Geometry: see drawing. Coordinates: mm, zero at the bounding-box minimum. A direction names the side the tool comes from. Coordinates: 2 decimals unless noted, no trailing zeros. Loops run counter-clockwise (first coordinate to the right, second up) from the corner with the lowest first, then second, coordinate; pieces in that order, holes last. Notation, with made-up numbers: (-26.5, 60) -> (11.5, 60) arc R25 ccw to (11.5, 80) -> close; hole circle Ø4 at (35, 16.5). An arc over 180 degrees is marked (long way). One line per item, written item: value. Start each with the question number.
Item 1: Set-up query: the marked faces 1, 2 and 3. Return all of +Z, -Z, +X, -X, +Y, -Y with unobstructed straight access to the full face (end or side cutting, diameter ignored); none if empty.
Item 2: Contact query for flat-ended pins moving along their axis: pin 1 Ø8 at (y, z) = (20, 15) entering from +X; pin 2 Ø2 at (x, z) = (54.5, 16) entering from +Y; pin 3 Ø6 at (y, z) = (36.5, 6) entering from +X; pin 4 Ø10 at (x, y) = (45, 14) entering from -Z. Output: stop coordinate, or through.
Item 3: Section query A-A on x = 10. Return loops of the section in (y, z), then the cut area to 3 significant figures.
Item 4: Section query D-D on x = 95.5. Return loops of the section in (y, z).
Item 5: Section query B-B on z = 3.25. Return loops of the section in (x, y), then the cut area to 3 significant figures.
Item 6: Section query C-C on z = 10. Return loops of the section in (x, y), then the cut area to 3 significant figures.
Item 7: Ray query, probe 1 along Z at (x, y) = (10, 1); probe 2 along Y at (x, z) = (13.5, 13.75); probe 3 along Y at (x, z) = (39, 14) (1 decimal). Return the intervals inside material, ascending. Write a range as from..to.
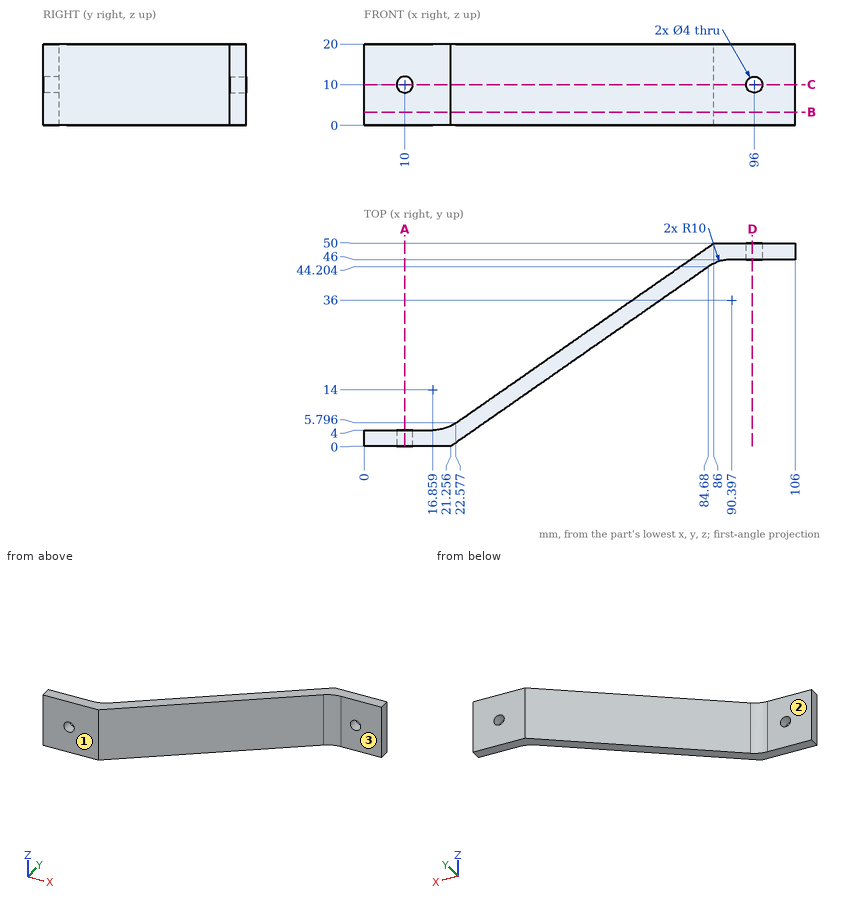
Reply:
1. face 1: +Z, -Z, +X, -X, -Y
1. face 2: +Z, -Z, -X, +Y
1. face 3: +Z, -Z, +X, -Y
2. pin 1: stops at x = 55.69
2. pin 2: stops at y = 28.74
2. pin 3: stops at x = 77.93
2. pin 4: stops at z = 0
3. outline: (0, 0) -> (4, 0) -> (4, 8) -> (0, 8) -> close; (0, 12) -> (4, 12) -> (4, 20) -> (0, 20) -> close
3. area: 64.0 mm²
4. outline: (46, 0) -> (50, 0) -> (50, 8.06) -> (46, 8.06) -> close; (46, 11.94) -> (50, 11.94) -> (50, 20) -> (46, 20) -> close
5. outline: (0, 0) -> (21.26, 0) -> (84.68, 44.2) arc R10 cw to (90.4, 46) -> (106, 46) -> (106, 50) -> (86, 50) -> (22.58, 5.8) arc R10 cw to (16.86, 4) -> (0, 4) -> close
5. area: 484 mm²
6. outline: (0, 0) -> (8, 0) -> (8, 4) -> (0, 4) -> close; (12, 0) -> (21.26, 0) -> (84.68, 44.2) arc R10 cw to (90.4, 46) -> (94, 46) -> (94, 50) -> (86, 50) -> (22.58, 5.8) arc R10 cw to (16.86, 4) -> (12, 4) -> close; (98, 46) -> (106, 46) -> (106, 50) -> (98, 50) -> close
6. area: 452 mm²
7. probe 1: z = 0..8, 12..20
7. probe 2: y = 0..4
7. probe 3: y = 12.4..17.2
